Build history of the part. All positions in model axes, mm. Round coordinates to 2 decimals unless told otherwise and drop trailing zeros. Write each loop counter-clockwise with the first axis right and the second up, starting at its lowest first coordinate (ties: lowest second). Pieces come first, ordered by that corner, then holes.
Item 1: Drop flat-ended pins along their axis: pin 1 Ø1.5 at (y, z) = (285, 1.5) entering from +X; pin 2 Ø3 at (x, z) = (72.5, 2) entering from -Y; pin 3 Ø1.5 at (x, z) = (98.5, 1.5) entering from +Y. Give the stop position or say it passes through.
Item 2: Band-saw the part on A-A, the plane y = 143. Write the cut outline in (x, z), then the cut area to 3 significant figures.
Item 3: Wall check: probe 1 along Y at (x, z) = (29, 3.1); probe 2 along X at (y, z) = (34, 4). Give the ranges that are in metal, low to high.
```python
from build123d import *

# Parameters (mm, degrees)
ESQUISSE1_W             = 100
ESQUISSE1_H             = 330
BOSS_EXTRU_1_DEPTH      = 5
ESQUISSE3_W             = 5
ESQUISSE3_H             = 10
ESQUISSE3_W_2           = 10
ESQUISSE3_H_2           = 3.898354104
ENL_V_MAT_EXTRU_1_DEPTH = 345.85504201


with BuildPart() as part:
    # Esquisse1 → Boss.-Extru.1 (new body)
    with BuildSketch(Plane.XY):
        with Locations((50, 165)):
            Rectangle(ESQUISSE1_W, ESQUISSE1_H)
    extrude(amount=BOSS_EXTRU_1_DEPTH)

    # Esquisse3 → Enlèv. mat.-Extru.1 (cut, through all)
    with BuildSketch(Plane.XY):
        with Locations((97.5, 325)):
            Rectangle(ESQUISSE3_W, ESQUISSE3_H)
        with Locations((97.5, 305)):
            Rectangle(ESQUISSE3_W, ESQUISSE3_H)
        with Locations((97.5, 285)):
            Rectangle(ESQUISSE3_W, ESQUISSE3_H)
        with Locations((97.5, 265)):
            Rectangle(ESQUISSE3_W, ESQUISSE3_H)
        with Locations((97.5, 245)):
            Rectangle(ESQUISSE3_W, ESQUISSE3_H)
        with Locations((97.5, 225)):
            Rectangle(ESQUISSE3_W, ESQUISSE3_H)
        with Locations((97.5, 205)):
            Rectangle(ESQUISSE3_W, ESQUISSE3_H)
        with Locations((97.5, 185)):
            Rectangle(ESQUISSE3_W, ESQUISSE3_H)
        with Locations((97.5, 165)):
            Rectangle(ESQUISSE3_W, ESQUISSE3_H)
        with Locations((97.5, 145)):
            Rectangle(ESQUISSE3_W, ESQUISSE3_H)
        with Locations((97.5, 125)):
            Rectangle(ESQUISSE3_W, ESQUISSE3_H)
        with Locations((97.5, 105)):
            Rectangle(ESQUISSE3_W, ESQUISSE3_H)
        with Locations((97.5, 85)):
            Rectangle(ESQUISSE3_W, ESQUISSE3_H)
        with Locations((97.5, 65)):
            Rectangle(ESQUISSE3_W, ESQUISSE3_H)
        Polygon((100, 50), (100, 40), (100, 0), (85, 0), (85, 3.898354104), (95, 3.898354104), (95, 40), (95, 50), align=None)
        with Locations((70, 1.949177052)):
            Rectangle(ESQUISSE3_W_2, ESQUISSE3_H_2)
        with Locations((50, 1.949177052)):
            Rectangle(ESQUISSE3_W_2, ESQUISSE3_H_2)
        with Locations((30, 1.949177052)):
            Rectangle(ESQUISSE3_W_2, ESQUISSE3_H_2)
        with Locations((10, 1.949177052)):
            Rectangle(ESQUISSE3_W_2, ESQUISSE3_H_2)
    extrude(amount=ENL_V_MAT_EXTRU_1_DEPTH, mode=Mode.SUBTRACT)


solid = part.part
```
Results:
1. pin 1: stops at x = 95
1. pin 2: stops at y = 3.9
1. pin 3: stops at y = 320
2. outline: (0, 0) - (95, 0) - (95, 5) - (0, 5) - close
2. area: 475 mm2
3. probe 1: y = 3.9 to 330
3. probe 2: x = 0 to 95
